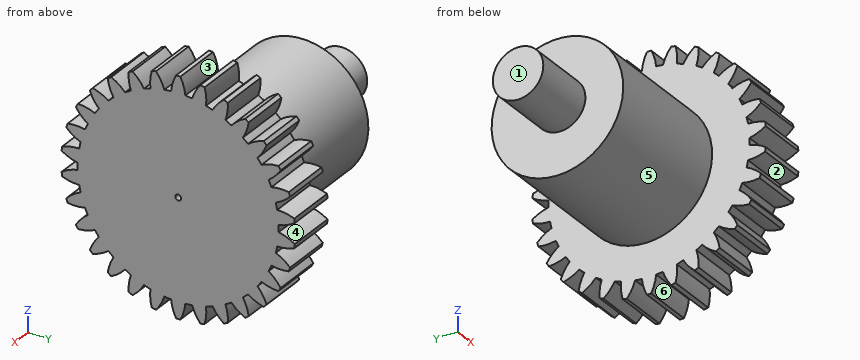
from build123d import *

# Parameters (mm, degrees)
BASPROSKE_W         = 7
BASPROSKE_H         = 16
TOOTHCUT_DEPTH      = 24.685438565
TEETHCUTS_COUNT     = 30
TEETHCUTS_ANGLE     = 348
BORSKE_R            = 0.4
BORE_DEPTH          = 50.0000508
SKETCH1_R           = 9
BOSS_EXTRUDE1_DEPTH = 19
SKETCH2_R           = 3.45
BOSS_EXTRUDE2_DEPTH = 9


with BuildPart() as part:
    # BasProSke → Base-Revolve (revolve)
    with BuildSketch(Plane(origin=(0, 0, 0), x_dir=(1, 0, 0), z_dir=(0, 1, 0)), mode=Mode.PRIVATE) as base_revolve_sk:
        with Locations((3.5, 8)):
            Rectangle(BASPROSKE_W, BASPROSKE_H)
    revolve(base_revolve_sk.sketch.rotate(Axis((-10, 0, 0), (1, 0, 0)), 180), axis=Axis((-10, 0, 0), (1, 0, 0)))

    # TooCutSke → ToothCut (cut, through all)
    with BuildSketch(Plane(origin=(0, 0, 0), x_dir=(0, 0, -1), z_dir=(1, 0, 0))):
        with BuildLine():
            ThreePointArc((0.466400716, 13.741086979), (0, 13.749), (-0.466400716, 13.741086979))
            ThreePointArc((-0.466400716, 13.741086979), (-0.819142092, 14.899954875), (-1.3974676, 15.964351834))
            ThreePointArc((-1.3974676, 15.964351834), (0, 16.0254), (1.3974676, 15.964351834))
            ThreePointArc((1.3974676, 15.964351834), (0.819142092, 14.899954875), (0.466400716, 13.741086979))
        make_face()
    toothcut = extrude(amount=TOOTHCUT_DEPTH, mode=Mode.SUBTRACT)

    # TeethCuts: ToothCut ×30 about axis
    teethcuts_axis = Axis((-10, 0, 0), (1, 0, 0))
    for i in range(1, TEETHCUTS_COUNT):
        add(toothcut.rotate(teethcuts_axis, i * TEETHCUTS_ANGLE / (TEETHCUTS_COUNT - 1)), mode=Mode.SUBTRACT)

    # BorSke → Bore (cut, symmetric)
    with BuildSketch(Plane(origin=(0, 0, 0), x_dir=(0, 0, -1), z_dir=(1, 0, 0))):
        with Locations(Location((0, 0, 0), (0, 0, 180))):
            Circle(BORSKE_R)
    extrude(amount=BORE_DEPTH, both=True, mode=Mode.SUBTRACT)

    # Sketch1 → Boss-Extrude1 (add)
    with BuildSketch(Plane.ZY):
        with Locations(Location((-0.138271535, 0.375341155, 0), (0, 0, 180))):
            Circle(SKETCH1_R)
    extrude(amount=BOSS_EXTRUDE1_DEPTH)

    # Sketch2 → Boss-Extrude2 (add)
    with BuildSketch(Plane.ZY.offset(19)):
        Circle(SKETCH2_R)
    extrude(amount=BOSS_EXTRUDE2_DEPTH)


solid = part.part
Work out the finished part from the listing and answer in its coordinate system (mm). Face numbers are marked on the shaded views. A direction names the side the tool comes from. Give positions to 0.01 mm unless a question says otherwise; leave off trailing zeros. Order: outer loops, then holes, each group sorted by start corner. A loop starts at its lowest first (then second) coordinate and runs counter-clockwise, first axis right, second up. Notation, with made-up numbers: (2, 47) -> (17, 47) arc R15 ccw to (17, 59) -> close; hole circle Ø6 at (5, 33.25). An arc over 180 degrees is marked (long way). Answer as a JSON object with one key per item and string values. Group by question number.
1. Section C-C on x = -21.5 is taken. Determine the outline of the cut face in (y, z), plus the area to 3 significant figures.
2. The mould has two halves that part along Z. Classify the marked faces 1, 2 and 3: released by +Z, released by -Z, zero draft, split by the parting line, or undercut.
3. Section B-B on z = -7 is taken. Determine the outline of the cut face in (x, y), plus the area to 3 significant figures.
4. A tool of negligible diameter and unlimited length cuts with its end or side. For the marked faces 4, 5 and 6, from which of +Z, -Z, +X, -X, +Y, -Y can it reach the whole face along a straight path? Write none if from no direction.
5. Section A-A on y = -5.5 is taken. Determine the outline of the cut face in (x, z), plus the area to 3 significant figures.
6. Section D-D on x = -17 is taken. Determine the outline of the cut face in (y, z), plus the area to 3 significant figures.
7. Consider line 1 along Y through (x, z) = (4, 0); line 2 along X through (y, z) = (6.5, -8.5); line 3 along X through (y, z) = (5, 4). Determine where each line is inside the solid, lowest interval first. Write a range as [from, to].
8. Flat-ended cylindrical pins translate along their axes: pin 1 Ø3 at (x, y) = (1.5, -2.5) entering from -Z; pin 2 Ø5 at (x, z) = (-8, -1.5) entering from +Y; pin 3 Ø5.5 at (y, z) = (4.5, 0) entering from -X; pin 4 Ø4 at (y, z) = (1, -11) entering from -X. Find the tip coordinate at first contact, or state that the pin passes through.
Result sheet:
{
 "1": {"outline": "circle Ø6.9 at (0, 0)", "area": "37.4 mm^2"},
 "2": {"face 1": "zero draft", "face 2": "undercut", "face 3": "released by +Z"},
 "3": {"outline": "(-19, -5.45) -> (0, -5.45) -> (0, -13.45) -> (7, -13.45) -> (7, 13.45) -> (0, 13.45) -> (0, 6.2) -> (-19, 6.2) -> close", "area": "410 mm^2"},
 "4": {"face 4": "+X, -X, +Y", "face 5": "-X", "face 6": "-Z, +X, -X"},
 "5": {"outline": "(-19, -6.96) -> (0, -6.96) -> (0, -14.05) -> (7, -14.05) -> (7, 14.05) -> (0, 14.05) -> (0, 6.68) -> (-19, 6.68) -> close", "area": "456 mm^2"},
 "6": {"outline": "circle Ø18 at (0.38, -0.14)", "area": "254 mm^2"},
 "7": {"line 1": "y = [-13.75, -0.4], [0.4, 13.75]", "line 2": "x = [0, 7]", "line 3": "x = [-19, 7]"},
 "8": {"pin 1": "stops at z = -15.71", "pin 2": "stops at y = 9.38", "pin 3": "stops at x = -28", "pin 4": "stops at x = -19"}
}
